Here's the drawing with two shaded views (mm, measured from the low corner). I have some questions. Round coordinates to 2 decimals unless told otherwise and drop trailing zeros. Loops run counter-clockwise (first coordinate to the right, second up) from the corner with the lowest first, then second, coordinate; pieces in that order, holes last.
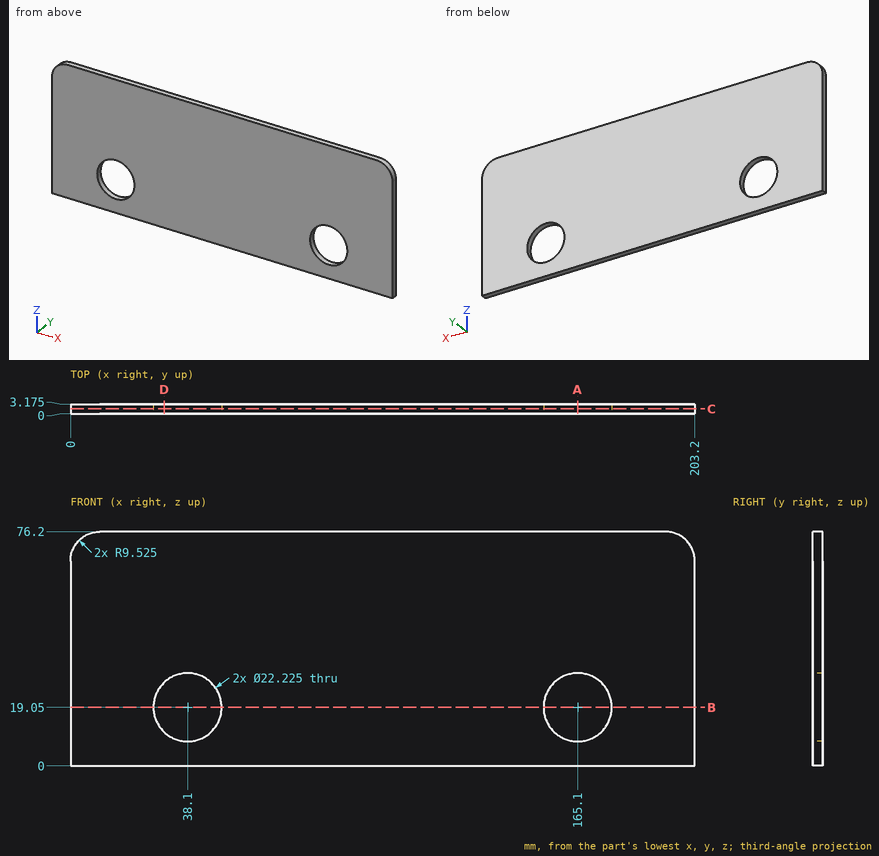
Item 1: If we section it at B-B, the plane z = 19.05: Please give me the cut outline in (x, y) (1 decimal).
Results list:
outline: (0, 0) - (27, 0) - (27, 3.2) - (0, 3.2) - close; (49.2, 0) - (154, 0) - (154, 3.2) - (49.2, 3.2) - close; (176.2, 0) - (203.2, 0) - (203.2, 3.2) - (176.2, 3.2) - close
Item 2: If we section it at C-C, the plane y = 1.6: Count the separate pieces of the cut face and the enclosed holes in it, then the cut area to 3 significant figures.
Results list:
separate pieces: 1
enclosed holes: 2
area: 14,700 mm2
Item 3: Will this pin go through, and if not, where does the flat tip stop? pin 1 (18 mm diameter, centred on x = 165.1, z = 19.05, fed in from -Y).
Results list:
pin 1: passes through
Item 4: If we section it at D-D, the plane x = 30.5: Please give me the cut outline in (y, z) (3 decimals).
Results list:
outline: (0, 0) - (3.175, 0) - (3.175, 10.943) - (0, 10.943) - close; (0, 27.157) - (3.175, 27.157) - (3.175, 76.2) - (0, 76.2) - close
Item 5: If we section it at A-A, the plane x = 165.1: Please give me the cut outline in (y, z) (1 decimal).
Results list:
outline: (0, 0) - (3.2, 0) - (3.2, 7.9) - (0, 7.9) - close; (0, 30.2) - (3.2, 30.2) - (3.2, 76.2) - (0, 76.2) - close
Item 6: If I drill on line 1 along X through (y, z) = (1.75, 19.05); line 2 along X through (y, z) = (0.8, 11.5); line 3 along Z through (x, y) = (168.5, 2.15), over which ranges is the centre line in solid material (lowest first)?
Results list:
line 1: x = 0 to 26.99, 49.21 to 153.99, 176.21 to 203.2
line 2: x = 0 to 29.95, 46.25 to 156.95, 173.25 to 203.2
line 3: z = 0 to 8.47, 29.63 to 76.2
